from build123d import *

# Parameters (mm, degrees)
SKETCH_1_W                  = 90
SKETCH_1_H                  = 60
EXTRUDE_1_DEPTH             = 30
HOLE_WIZARD_1_D             = 10
HOLE_WIZARD_M6_1_AT_2_COUNT = 2
HOLE_WIZARD_M6_1_AT_2_PITCH = 50
CUT_EXTRUDE_1_DEPTH         = 62.846584384
HOLE_WIZARD_M6_2_D          = 5
HOLE_WIZARD_M6_2_DEPTH      = 15
HOLE_WIZARD_M6_2_TIP        = 1.502151548
CUT_EXTRUDE_2_DEPTH         = 100.498743771


with BuildPart() as part:
    # 草图1 → 凸台-拉伸1 (new body)
    with BuildSketch(Plane(origin=(0, 0, 0), x_dir=(1, 0, 0), z_dir=(0, 1, 0))):
        Rectangle(SKETCH_1_W, SKETCH_1_H)
    extrude(amount=EXTRUDE_1_DEPTH)

    # 孔1 (through all)
    with Locations(Plane.XY.offset(30)):
        with Locations((0, 18)):
            Hole(HOLE_WIZARD_1_D / 2)

    # 草图4 → M6 螺纹孔1 (revolve, cut)
    with BuildSketch(Plane(origin=(-25, 18, 30), x_dir=(0, -1, 0), z_dir=(1, 0, 0))):
        Polygon((0, 0), (0, 16.502151548), (2.5, 15), (2.5, 0), align=None)
    hole_wizard_m6_1 = revolve(axis=Axis((-25, 18, 36.35), (0, 0, -1)), mode=Mode.SUBTRACT)

    # M6 螺纹孔1 at 2: M6 螺纹孔1 ×2
    with Locations(*[(i * HOLE_WIZARD_M6_1_AT_2_PITCH, 0, 0) for i in range(1, HOLE_WIZARD_M6_1_AT_2_COUNT)]):
        add(hole_wizard_m6_1, mode=Mode.SUBTRACT)

    # 镜向1: M6 螺纹孔1 across plane
    add(hole_wizard_m6_1.mirror(Plane.XY), mode=Mode.SUBTRACT)

    # 镜向1 copy 1 sketch → 镜向1 copy 1 (revolve, cut)
    with BuildSketch(Plane(origin=(25, 18, -30), x_dir=(0, -1, 0), z_dir=(1, 0, 0))):
        Polygon((0, 0), (0, -16.502151548), (2.5, -15), (2.5, 0), align=None)
    revolve(axis=Axis((25, 18, -36.35), (0, 0, -1)), mode=Mode.SUBTRACT)

    # 草图6 → 切除-拉伸1 (cut, through all)
    with BuildSketch(Plane(origin=(0, 30, 0), x_dir=(1, 0, 0), z_dir=(0, 1, 0))):
        with BuildLine():
            Line((-26, -18), (26, -18))
            ThreePointArc((26, -18), (28.828427125, -16.828427125), (30, -14))
            Line((30, -14), (30, 14))
            ThreePointArc((30, 14), (28.828427125, 16.828427125), (26, 18))
            Line((26, 18), (-26, 18))
            ThreePointArc((-26, 18), (-28.828427125, 16.828427125), (-30, 14))
            Line((-30, 14), (-30, -14))
            ThreePointArc((-30, -14), (-28.828427125, -16.828427125), (-26, -18))
        make_face()
    extrude(amount=-CUT_EXTRUDE_1_DEPTH, mode=Mode.SUBTRACT)

    # M6 螺纹孔2
    with Locations(Plane(origin=(0, 0, 0), x_dir=(-1, 0, 0), z_dir=(0, -1, 0))):
        with Locations((-39, -24), (39, -24), (39, 24), (-39, 24)):
            Hole(HOLE_WIZARD_M6_2_D / 2, depth=HOLE_WIZARD_M6_2_DEPTH)
            with Locations((0, 0, -(HOLE_WIZARD_M6_2_DEPTH + HOLE_WIZARD_M6_2_TIP / 2))):  # 118° drill point
                Cone(0, HOLE_WIZARD_M6_2_D / 2, HOLE_WIZARD_M6_2_TIP, mode=Mode.SUBTRACT)

    # 草图9 → 切除-拉伸2 (cut, through all)
    with BuildSketch(Plane(origin=(45, 0, 0), x_dir=(0, 0, -1), z_dir=(1, 0, 0))):
        with BuildLine():
            Line((-14, 6), (14, 6))
            ThreePointArc((14, 6), (16.828427125, 7.171572875), (18, 10))
            Line((18, 10), (18, 20))
            ThreePointArc((18, 20), (16.828427125, 22.828427125), (14, 24))
            Line((14, 24), (-14, 24))
            ThreePointArc((-14, 24), (-16.828427125, 22.828427125), (-18, 20))
            Line((-18, 20), (-18, 10))
            ThreePointArc((-18, 10), (-16.828427125, 7.171572875), (-14, 6))
        make_face()
    extrude(amount=-CUT_EXTRUDE_2_DEPTH, mode=Mode.SUBTRACT)


solid = part.part
Can you work these out from the model? Positions are in its coordinate system, mm. A direction names the side the tool comes from. Coordinates: 2 decimals unless noted, no trailing zeros. Write each loop counter-clockwise with the first axis right and the second up, starting at its lowest first coordinate (ties: lowest second). Pieces come first, ordered by that corner, then holes.
Q1. Which directions (+Z, -Z, +X, -X, +Y, -Y) give clear straight access to the entire face, cutting with the end or side of a thin tool? Please do faces 1 (the face through (38, 6, 0)), 2 (the face through (40.34, 7.6, 21.89)), 3 (the face through (1.08, 13.12, 23.92)), 4 (the face through (1, 11, -18)), 5 (the face through (28.859, 26.256, -16.797)).
Results found:
face 1: +X, -X
face 2: -Y
face 3: +Z, -Z
face 4: none
face 5: +Y, -Y
Q2. Please list where these lines run through material, in increasing order: L1, parallel to X at y = 10, z = -24; L2, parallel to X at y = 3, z = 9.5; L3, parallel to Y at x = 39, z = 1.5.
Results found:
L1: x = -45 to -41.5, -36.5 to 36.5, 41.5 to 45
L2: x = -45 to -30, 30 to 45
L3: y = 0 to 6, 24 to 30
Q3. Imagine slicing it at C-C, the plane y = 4.5. List the corners of the cut face in (x, z) for me.
Results found:
outline: (-45, -30) - (45, -30) - (45, 30) - (-45, 30) - close; hole circle Ø5 at (-39, -24); hole circle Ø5 at (-39, 24); hole (-30, -14) arc R4 ccw to (-26, -18) - (26, -18) arc R4 ccw to (30, -14) - (30, 14) arc R4 ccw to (26, 18) - (-26, 18) arc R4 ccw to (-30, 14) - close; hole circle Ø5 at (39, -24); hole circle Ø5 at (39, 24)
Q4. If we mould it in two halves opening along X, with no side actions, what happens to faces 6 (the face through (-45, 25, 0)), 7 (the face through (-26.69, 19.84, 24.08)), 8 (the face through (-37.478, 7.141, -16.797))? For each: +X half, -X half, draft (parallel to the pull), parting line (faces both ways), or undercut.
Results found:
face 6: -X half
face 7: undercut
face 8: draft
Q5. Imagine slicing it at D-D, the plane y = 18. Count the separate pieces of the cut face and the enclosed holes in it, plus the area to 3 significant figures.
Results found:
separate pieces: 8
enclosed holes: 0
area: 1,680 mm2
Q6. Imagine slicing it at B-B, the plane x = 0. List the corners of the cut face in (y, z) for me.
Results found:
outline: (0, -30) - (13, -30) - (13, -18) - (0, -18) - close; (0, 18) - (13, 18) - (13, 30) - (0, 30) - close; (23, -30) - (30, -30) - (30, -18) - (23, -18) - close; (23, 18) - (30, 18) - (30, 30) - (23, 30) - close
Q7. Imagine slicing it at A-A, the plane z = -8. List the corners of the cut face in (x, y) for me, plus the area to 3 significant figures.
Results found:
outline: (-45, 0) - (-30, 0) - (-30, 6) - (-45, 6) - close; (-45, 24) - (-30, 24) - (-30, 30) - (-45, 30) - close; (30, 0) - (45, 0) - (45, 6) - (30, 6) - close; (30, 24) - (45, 24) - (45, 30) - (30, 30) - close
area: 360 mm2
